Study the drawing (mm; zero at the part's minimum x, y, z) and answer. A direction names the side the tool comes from. Give positions to 0.01 mm unless a question says otherwise; leave off trailing zeros. Write each loop counter-clockwise with the first axis right and the second up, starting at its lowest first coordinate (ties: lowest second). Pieces come first, ordered by that corner, then holes.
1) Find section D-D (y = 37). Determine the outline of the cut face in (x, z).
2) Find section B-B (z = 19). Determine the outline of the cut face in (x, y), plus the area to 3 significant figures.
3) A tool of negligible diameter and unlimited length cuts with its end or side. For the marked faces 4, 5 and 6, from which of +Z, -Z, +X, -X, +Y, -Y can it reach the whole face along a straight path? Write none if from no direction.
4) Find section A-A (y = 42.5). Determine the outline of the cut face in (x, z), plus the area to 3 significant figures.
5) Given pin 1 Ø11.5 at (x, z) = (52.5, 4.5) entering from +Y; pin 2 Ø2 at (x, z) = (42, 39) entering from -Y; pin 3 Ø1.5 at (x, z) = (17, 7) entering from +Y; pin 4 Ø8 at (y, z) = (18.5, 40) entering from +X, each flat-ended and moving along its own axis, determine where each tip first touches the part or whether it passes through.
6) Find section C-C (x = 71). Determine the outline of the cut face in (y, z) (1 decimal), plus the area to 3 significant figures.
7) Determine the mould class of the marked faces 1, 2 and 3 for opening direction X: pulls with the +X half, pulls with the -X half, needs draft (parallel to the pull), parting line crosses it, or undercut.
8) Straight lines are drawn through the part: probe 1 along X at (y, z) = (5, 21); probe 2 along Y at (x, z) = (46.5, 36) (1 decimal); probe 3 along Y at (x, z) = (9.5, 3.5). For each, find the intervals that lie inside material, in ascending order.
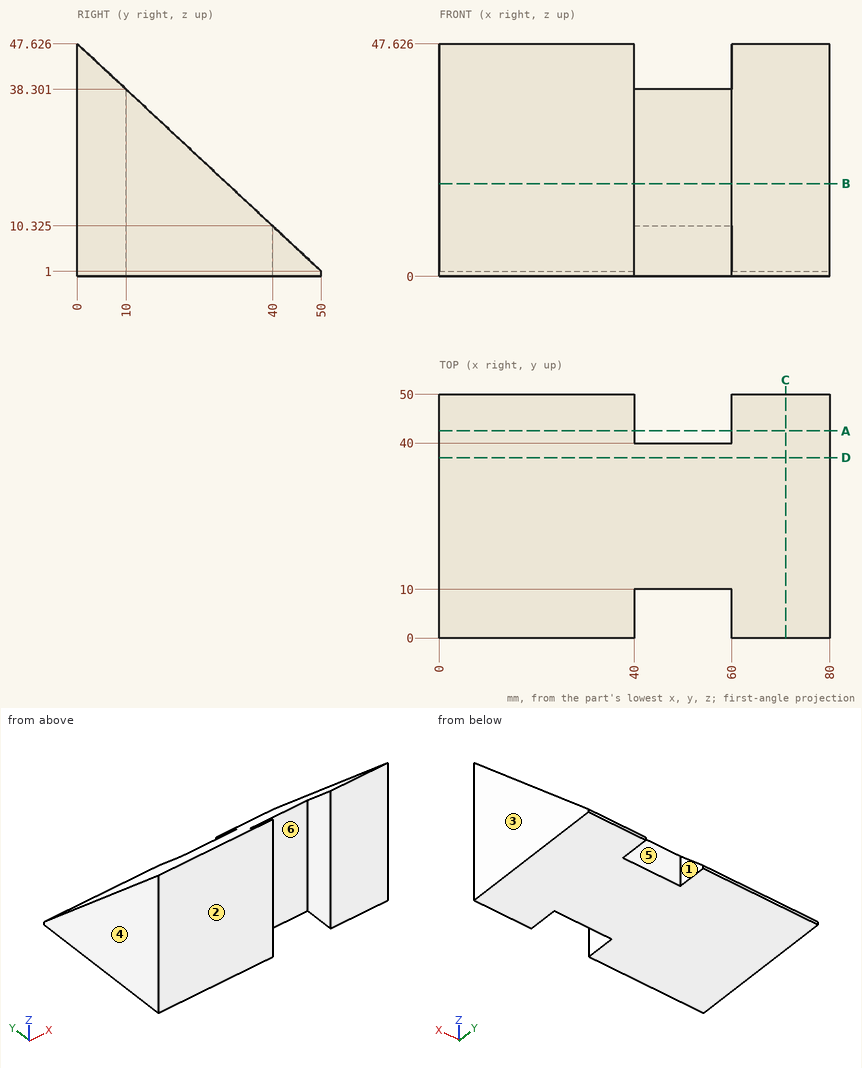
Results:
1. outline: (0, 0) - (80, 0) - (80, 13.12) - (0, 13.12) - close
2. outline: (0, 0) - (40, 0) - (40, 10) - (60, 10) - (60, 0) - (80, 0) - (80, 30.7) - (0, 30.7) - close
2. area: 2,260 mm2
3. face 4: +Z, -Z, -X, +Y, -Y
3. face 5: +Z, -Z, +Y
3. face 6: +Z, -Z, -Y
4. outline: (0, 0) - (40, 0) - (40, 7.99) - (0, 7.99) - close; (60, 0) - (80, 0) - (80, 7.99) - (60, 7.99) - close
4. area: 480 mm2
5. pin 1: stops at y = 40
5. pin 2: stops at y = 10
5. pin 3: stops at y = 44.37
5. pin 4: passes through
6. outline: (0, 0) - (50, 0) - (50, 1) - (0, 47.6) - close
6. area: 1,220 mm2
7. face 1: undercut
7. face 2: needs draft
7. face 3: pulls with the +X half
8. probe 1: x = 0 to 40, 60 to 80
8. probe 2: y = 10 to 12.5
8. probe 3: y = 0 to 47.32
